Read the model definition and answer for the solid it produces. Units are mm, in the model's axes. Round coordinates to 2 decimals unless told otherwise and drop trailing zeros. Order: outer loops, then holes, each group sorted by start corner. A loop starts at its lowest first (then second) coordinate and runs counter-clockwise, first axis right, second up. Notation, with made-up numbers: (56.25, 81) -> (70.25, 81) arc R23 ccw to (70.25, 105) -> close; hole circle Ø6 at (64, 73). An arc over 180 degrees is marked (long way). Answer as a JSON object with one key per item and string values. Group by question number.
Item 1: Section A-A, the plane x = 1536 is taken. Write down the section's boundary in (y, z).
Item 2: Consider probe 1 along Z at (x, y) = (1416.5, 3); probe 2 along Z at (x, y) = (1201, -1.5); probe 3 along Y at (x, z) = (2048, -18.75). Determine where each line is inside the solid, lowest interval first. Write a range as from..to.
Item 3: Given P1, Ø7, axis at x = 2048, y = 0, coming from the +Z side; P2, Ø5, axis at x = 449.5, y = -21.5, coming from the +Z side; P3, Ø5, axis at y = -21.5, z = 15, coming from the +X side; P4, Ø12, axis at x = 729, z = -11, coming from the -Y side, each flat-ended and moving along its own axis, determine where each tip first touches the part or whether it passes through.
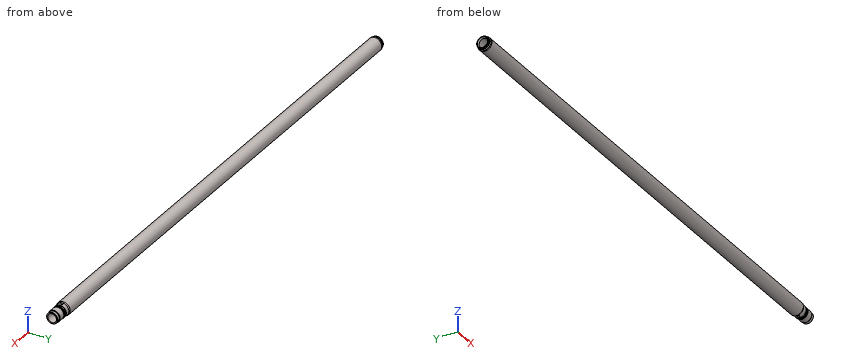
from build123d import *

# Parameters (mm, degrees)
SKETCH2_R          = 4.5
CUT_EXTRUDE1_DEPTH = 50


with BuildPart() as part:
    # Sketch1 → Base-Revolve (revolve)
    with BuildSketch(Plane.XY):
        with BuildLine():
            Line((0, 21), (0, 23.5))
            Line((0, 23.5), (0.5, 24))
            Line((0.5, 24), (5, 24))
            Line((5, 24), (5, 24.75))
            Line((5, 24.75), (7.5, 24.75))
            Line((7.5, 24.75), (11.830127019, 27.25))
            Line((11.830127019, 27.25), (17, 27.25))
            Line((17, 27.25), (17, 27.5))
            Line((17, 27.5), (2038.669872981, 27.5))
            Line((2038.669872981, 27.5), (2043, 25))
            Line((2043, 25), (2059.5, 25))
            ThreePointArc((2059.5, 25), (2059.853553391, 24.853553391), (2060, 24.5))
            Line((2060, 24.5), (2060, 23.5))
            Line((2060, 23.5), (2066, 23.5))
            Line((2066, 23.5), (2066, 24.5))
            ThreePointArc((2066, 24.5), (2066.146446609, 24.853553391), (2066.5, 25))
            Line((2066.5, 25), (2068, 25))
            Line((2068, 25), (2069, 24.422649731))
            Line((2069, 24.422649731), (2069, 23.75))
            ThreePointArc((2069, 23.75), (2069.292893219, 23.042893219), (2070, 22.75))
            Line((2070, 22.75), (2072, 22.75))
            Line((2072, 22.75), (2074.453263132, 24))
            Line((2074.453263132, 24), (2098.401923789, 24))
            Line((2098.401923789, 24), (2101, 22.5))
            Line((2101, 22.5), (2111, 22.5))
            Line((2111, 22.5), (2112, 21.922649731))
            Line((2112, 21.922649731), (2112, 17.5))
            Line((2112, 17.5), (6.062177826, 17.5))
            Line((6.062177826, 17.5), (0, 21))
        make_face()
    revolve(axis=Axis((0, 0, 0), (1, 0, 0)))

    # Sketch2 → Cut-Extrude1 (cut, symmetric)
    with BuildSketch(Plane.XY):
        with Locations((2048, 0)):
            Circle(SKETCH2_R)
    extrude(amount=CUT_EXTRUDE1_DEPTH, both=True, mode=Mode.SUBTRACT)


solid = part.part
Values found:
{
 "1": {"outline": "circle Ø55 at (0, 0); hole circle Ø35 at (0, 0)"},
 "2": {"probe 1": "-27.34..-17.24, 17.24..27.34", "probe 2": "-27.46..-17.44, 17.44..27.46", "probe 3": "-16.54..-4.5, 4.5..16.54"},
 "3": {"P1": "through", "P2": "z = 19.88", "P3": "x = 2098.89", "P4": "y = -27.04"}
}
